Geometry: final body of the model. Coordinates: model frame, mm. Face numbers are marked on the shaded views. A direction names the side the tool comes from. Give positions to 0.01 mm unless a question says otherwise; leave off trailing zeros. Write each loop counter-clockwise with the first axis right and the second up, starting at its lowest first coordinate (ties: lowest second). Pieces come first, ordered by that corner, then holes. Notation, with made-up numbers: (-15.75, 73.5) -> (36.25, 73.5) arc R22 cw to (36.25, 107.5) -> close; hole circle Ø11 at (-10.5, 16). An arc over 180 degrees is marked (long way). Use CSV: the item, a comma, the result in double quotes. Start each with the question number.
1) Draft query along X for the marked faces 5, 6 and 7. Return one class per face: pulls with the +X half, pulls with the -X half, needs draft (parallel to the pull), parting line crosses it, or undercut.
2) Section C-C (y = -40). Output: boundary loops of the cut face in (x, z), plus the area to 3 significant figures.
3) Material intervals for line 1 (X direction, y = -84, z = 70); line 2 (Y direction, x = -18, z = 62); line 3 (Z direction, x = 32, y = -72), sorted ascending. Write a range as [from, to].
4) Section D-D (x = -31.5). Output: boundary loops of the cut face in (y, z).
5) Set-up query: the marked faces 1, 2, 3 and 4. Return all of +Z, -Z, +X, -X, +Y, -Y with unobstructed straight access to the full face (end or side cutting, diameter ignored); none if empty.
6) Section A-A (y = -90). Output: boundary loops of the cut face in (x, z).
7) Contact query for flat-ended pins moving along their axis: P1, Ø12, axis at x = -4, y = -62, coming from the -Z side; P2, Ø15, axis at y = -32.5, z = 4, coming from the +X side; P3, Ø3, axis at y = -21, z = -5, coming from the -X side; P4, Ø8, axis at x = -19.5, z = 43, coming from the -Y side. Output: stop coordinate, or through.
8) Section B-B (z = 45). Output: boundary loops of the cut face in (x, y), plus the area to 3 significant figures.
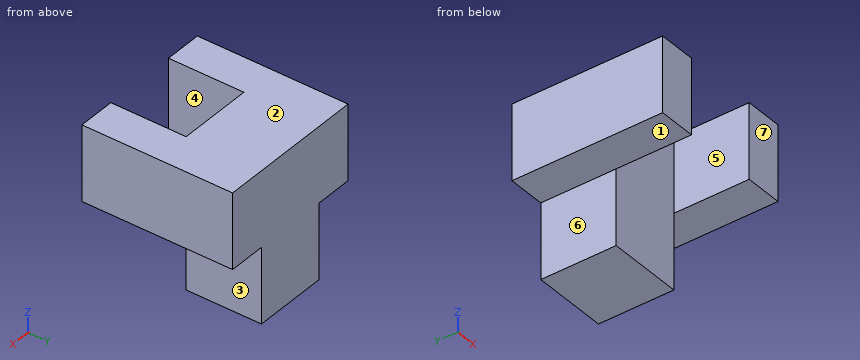
```python
from build123d import *

# Parameters (mm, degrees)
F0_W     = 101.6
F0_H     = 50.8
F1_DEPTH = 50.8
F2_W     = 25.4
F2_H     = 101.6
F3_DEPTH = 50.8
F4_W     = 50.800001
F4_H     = 50.8
F5_DEPTH = 50.8


with BuildPart() as f1:
    # F0 (on Front) → F1 (new body)
    with BuildSketch(Plane.XZ):
        with Locations((-7.620003, 52.950555)):
            Rectangle(F0_W, F0_H)
    extrude(amount=F1_DEPTH)

    # F2 (on face) → F3 (join)
    with BuildSketch(Plane.XY.offset(78.350555)):
        with Locations((-45.720003, -50.8)):
            Rectangle(F2_W, F2_H)
        with Locations((30.479997, -50.8)):
            Rectangle(F2_W, F2_H)
    extrude(amount=-F3_DEPTH)

    # F4 (on face) → F5 (join)
    with BuildSketch(Plane(origin=(0, 0, 27.550555), x_dir=(1, 0, 0), z_dir=(0, 0, -1))):
        with Locations((-7.620002, 25.4)):
            Rectangle(F4_W, F4_H)
    extrude(amount=F5_DEPTH)


solid = f1.part
```
Answers follow:
1,face 5,"undercut"
1,face 6,"pulls with the -X half"
1,face 7,"needs draft"
2,outline,"(-58.42, 27.55) -> (-33.02, 27.55) -> (-33.02, -23.25) -> (17.78, -23.25) -> (17.78, 27.55) -> (43.18, 27.55) -> (43.18, 78.35) -> (-58.42, 78.35) -> close"
2,area,"7,740 mm^2"
3,line 1,"x = [-58.42, -33.02], [17.78, 43.18]"
3,line 2,"y = [-50.8, 0]"
3,line 3,"z = [27.55, 78.35]"
4,outline,"(-50.8, -23.25) -> (0, -23.25) -> (0, 78.35) -> (-50.8, 78.35) -> close"
5,face 1,"-Z, -X, +Y, -Y"
5,face 2,"+Z, +X, -X, +Y, -Y"
5,face 3,"-Z, +X, +Y, -Y"
5,face 4,"+Z, -Z, -Y"
6,outline,"(-58.42, 27.55) -> (-33.02, 27.55) -> (-33.02, 78.35) -> (-58.42, 78.35) -> close; (17.78, 27.55) -> (43.18, 27.55) -> (43.18, 78.35) -> (17.78, 78.35) -> close"
7,P1,"passes through"
7,P2,"stops at x = 17.78"
7,P3,"stops at x = -33.02"
7,P4,"stops at y = -50.8"
8,outline,"(-58.42, -101.6) -> (-33.02, -101.6) -> (-33.02, -50.8) -> (17.78, -50.8) -> (17.78, -101.6) -> (43.18, -101.6) -> (43.18, 0) -> (-58.42, 0) -> close"
8,area,"7,740 mm^2"
